The model under review builds one solid part; all positions refer to its coordinate system, in mm. Give positions to 0.01 mm unless a question says otherwise; leave off trailing zeros. Order: outer loops, then holes, each group sorted by start corner. A loop starts at its lowest first (then second) coordinate and runs counter-clockwise, first axis right, second up. Notation, with made-up numbers: (-2.5, -11.5) - (32.5, -11.5) arc R10 ccw to (32.5, -6.5) - close; hole circle Ø6 at (49, 40). An arc over 180 degrees is marked (long way). Use CSV: the item, a comma, the result in double quotes.
```python
from build123d import *

# Parameters (mm, degrees)
PLATE_START      = -40
SKETCH1_W        = 245
SKETCH1_H        = 10
PLATE_DEPTH      = 305
EXTRUDE_START    = -12
SKETCH2_R        = 3.3
EXTRUDE_H0_DEPTH = 14
SKETCH3_R        = 3.3
EXTRUDE_H1_DEPTH = 14
SKETCH4_R        = 3.3
EXTRUDE_H2_DEPTH = 14
SKETCH5_R        = 3.3
EXTRUDE_H3_DEPTH = 14


with BuildPart() as part:
    # Sketch1 → plate (new body)
    with BuildSketch(Plane(origin=(0, 0, 0), x_dir=(0, 0, -1), z_dir=(1, 0, 0)).offset(PLATE_START)):
        with Locations((-12.5, -5)):
            Rectangle(SKETCH1_W, SKETCH1_H)
    extrude(amount=PLATE_DEPTH)


with BuildPart() as body_2:
    # Sketch2 → Extrude h0 (new body)
    with BuildSketch(Plane(origin=(0, 0, 0), x_dir=(1, 0, 0), z_dir=(0, 1, 0)).offset(EXTRUDE_START)):
        with Locations(Location((-30, 100, 0), (0, 0, 270))):
            Circle(SKETCH2_R)
    extrude(amount=EXTRUDE_H0_DEPTH)


with BuildPart() as part_1:
    add(part.part)

    # Combine1: cut body 2
    add(body_2.part, mode=Mode.SUBTRACT)


with BuildPart() as body_2_2:
    # Sketch3 → Extrude h1 (new body)
    with BuildSketch(Plane(origin=(0, 0, 0), x_dir=(1, 0, 0), z_dir=(0, 1, 0)).offset(EXTRUDE_START)):
        with Locations(Location((-30, -125, 0), (0, 0, 270))):
            Circle(SKETCH3_R)
    extrude(amount=EXTRUDE_H1_DEPTH)


with BuildPart() as part_2:
    add(part_1.part)

    # Combine2: cut body 2 2
    add(body_2_2.part, mode=Mode.SUBTRACT)


with BuildPart() as body_2_3:
    # Sketch4 → Extrude h2 (new body)
    with BuildSketch(Plane(origin=(0, 0, 0), x_dir=(1, 0, 0), z_dir=(0, 1, 0)).offset(EXTRUDE_START)):
        with Locations(Location((255, 100, 0), (0, 0, 270))):
            Circle(SKETCH4_R)
    extrude(amount=EXTRUDE_H2_DEPTH)


with BuildPart() as part_3:
    add(part_2.part)

    # Combine3: cut body 2 3
    add(body_2_3.part, mode=Mode.SUBTRACT)


with BuildPart() as body_2_4:
    # Sketch5 → Extrude h3 (new body)
    with BuildSketch(Plane(origin=(0, 0, 0), x_dir=(1, 0, 0), z_dir=(0, 1, 0)).offset(EXTRUDE_START)):
        with Locations(Location((255, -125, 0), (0, 0, 270))):
            Circle(SKETCH5_R)
    extrude(amount=EXTRUDE_H3_DEPTH)


with BuildPart() as part_4:
    add(part_3.part)

    # Combine4: cut body 2 4
    add(body_2_4.part, mode=Mode.SUBTRACT)


solid = part_4.part
```
Item 1: Mouldability with a two-part tool opening along X and no side actions: class faces 1 (the face through (252.992, -5.07, 122.381)), 2 (the face through (-40, -5, 14)), 3 (the face through (110, 0, 14)) as pulls with the +X half, pulls with the -X half, needs draft (parallel to the pull), parting line crosses it, or undercut.
Results list:
face 1,"undercut"
face 2,"pulls with the -X half"
face 3,"needs draft"
Item 2: Clearance check with flat-ended pins moving along their axes: pin 1 (12 mm diameter, centred on x = 159, z = 46, fed in from +Y); pin 2 (6 mm diameter, centred on x = -30, z = 125, fed in from -Y). State where each tip first meets the part, or that it passes through.
Results list:
pin 1,"stops at y = 0"
pin 2,"passes through"
Item 3: Wall thickness on L1, parallel to X at y = -5.75, z = 125; L2, parallel to Z at x = -30, y = -7.25: over which ranges is each line inside the solid? List them lowest first.
Results list:
L1,"x = -40 to -33.3, -26.7 to 251.7, 258.3 to 265"
L2,"z = -110 to -103.3, -96.7 to 121.7, 128.3 to 135"
Item 4: Take a section at B-B, the plane z = -100. Give the boundary of the cut face in (x, y).
Results list:
outline,"(-40, -10) - (-33.3, -10) - (-33.3, 0) - (-40, 0) - close; (-26.7, -10) - (251.7, -10) - (251.7, 0) - (-26.7, 0) - close; (258.3, -10) - (265, -10) - (265, 0) - (258.3, 0) - close"
Item 5: Take a section at A-A, the plane x = -30. Give the boundary of the cut face in (y, z), and give its area (3 significant figures).
Results list:
outline,"(-10, -110) - (0, -110) - (0, -103.3) - (-10, -103.3) - close; (-10, -96.7) - (0, -96.7) - (0, 121.7) - (-10, 121.7) - close; (-10, 128.3) - (0, 128.3) - (0, 135) - (-10, 135) - close"
area,"2,320 mm2"
